```python
from build123d import *

# Parameters (mm, degrees)
BOSS_EXTRUDE1_DEPTH  = 3.175
M3_CLEARANCE_HOLE1_D = 3.2


with BuildPart() as part:
    # Sketch1 → Boss-Extrude1 (new body)
    with BuildSketch(Plane(origin=(0, 0, 0), x_dir=(1, 0, 0), z_dir=(0, 1, 0))):
        with BuildLine():
            Line((-95.25, 12.7), (95.25, 12.7))
            ThreePointArc((95.25, 12.7), (107.95, 0), (95.25, -12.7))
            Line((95.25, -12.7), (-95.25, -12.7))
            ThreePointArc((-95.25, -12.7), (-107.95, 0), (-95.25, 12.7))
        make_face()
    extrude(amount=BOSS_EXTRUDE1_DEPTH)

    # M3 Clearance Hole1 (through all)
    with Locations(Plane(origin=(0, 3.175, 0), x_dir=(1, 0, 0), z_dir=(0, 1, 0))):
        with Locations((-95.25, 0), (0, 0), (95.25, 0)):
            Hole(M3_CLEARANCE_HOLE1_D / 2)


solid = part.part
```
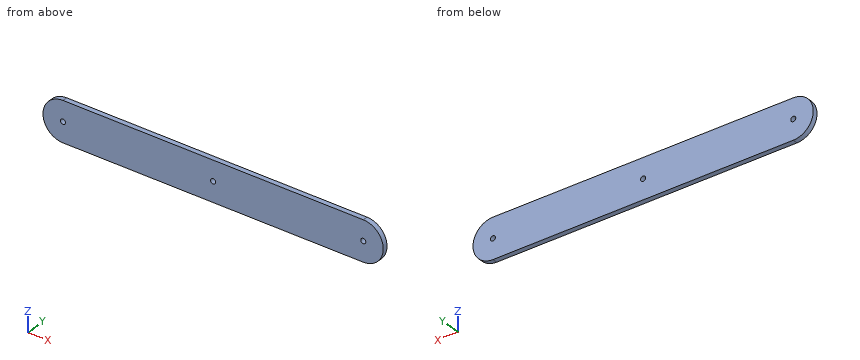
The listing builds one solid part. Answer for the finished solid, in the listing's coordinates (mm). Coordinates: 2 decimals unless noted, no trailing zeros. Order: outer loops, then holes, each group sorted by start corner. A loop starts at its lowest first (then second) coordinate and runs counter-clockwise, first axis right, second up. Notation, with made-up numbers: M 58,46.25 L 106,46.25 A27 cw 106,65.25 Z; hole C 28.25,51.25 d2. An arc over 180 degrees is marked long. Answer as a JSON object with one key per item and string values. Group by question number.
1. Straight lines are drawn through the part: line 1 (X direction, y = 1.65, z = -0.25); line 2 (Z direction, x = 95.25, y = 1.25); line 3 (X direction, y = 1.95, z = -7). For each, find the intervals that lie inside material, in ascending order.
2. Section B-B on z = 9.75 is taken. Write down the section's boundary in (x, y) (3 decimals).
3. Flat-ended cylindrical pins translate along their axes: P1, Ø1, axis at y = 2.5, z = -1, coming from the +X side; P2, Ø5, axis at x = 76, z = -9, coming from the -Y side. Find the tip coordinate at first contact, or state that the pin passes through.
4. Section A-A on y = 1.85 is taken. Write down the section's boundary in (x, z).
Values follow:
{
 "1": {"line 1": "-107.95 to -96.83, -93.67 to -1.58, 1.58 to 93.67, 96.83 to 107.95", "line 2": "-12.7 to -1.6, 1.6 to 12.7", "line 3": "-105.85 to 105.85"},
 "2": {"outline": "M -103.388,0 L 103.388,0 L 103.388,3.175 L -103.388,3.175 Z"},
 "3": {"P1": "x = 107.94", "P2": "y = 0"},
 "4": {"outline": "M -95.25,-12.7 L 95.25,-12.7 A12.7 ccw 95.25,12.7 L -95.25,12.7 A12.7 ccw Z; hole C -95.25,0 d3.2; hole C 0,0 d3.2; hole C 95.25,0 d3.2"}
}
